Autodesk Inventor part; units mm, degrees
ref_plane "Plan de construction1" through (0, 0, 5) normal (0, 0, 1) x (1, 0, 0)
ref_plane "YZ Plane" through (0, 0, 0) normal (1, 0, 0) x (0, 1, 0)
ref_plane "XZ Plane" through (0, 0, 0) normal (0, 1, 0) x (-1, 0, 0)
sketch "Esquisse1" plane through (0, 0, 0) normal (0, 1, 0) x (-1, 0, 0)
  arc A0 (0, -5) -> (0, 5) centre (0, 0) ccw
  line L0 (0, 5) -> (0, -5)
  dimension "d1" = 5
revolve "Révolution1" add sketch "Esquisse1" angle 360 about axis through (0, 0, 5) along (0, 0, -1)
ref_plane "Plan de construction1" through (0, 0, 5) normal (0, 0, 1) x (1, 0, 0)
sketch "Esquisse2" plane through (0, 0, 5) normal (0, 0, 1) x (1, 0, 0)
  circle A0 centre (0, 0) radius 2.5
  dimension "d4" = 5
extrude "Extrusion1" cut sketch "Esquisse2" against normal blind 0.5
sketch "Esquisse3" plane through (0, 0, 4.5) normal (0, 0, 1) x (1, 0, 0)
  circle A0 centre (0, 0) radius 2.1794
hole "Perçage1" at (0, 0, 4.5) direction (0, 0, -1) diameter 3.242 depth 5.5 tip angle 118
properties part number "boule_serrage_main" material "Plastique ABS"
Geometry check sheet. Reference: the model listing, model coordinates, mm. Round coordinates to 2 decimals unless told otherwise and drop trailing zeros. Write each loop counter-clockwise with the first axis right and the second up, starting at its lowest first coordinate (ties: lowest second). Pieces come first, ordered by that corner, then holes. Notation, with made-up numbers: (39.5, 41) - (66.5, 41) arc R15 ccw to (66.5, 60) - close; hole circle Ø1 at (55, 58). An arc over 180 degrees is marked (long way). Write each question's results on one line, items separated by ' | '.
(1) Sectioned sample at B-B, the plane x = 3. Enter the section's corners in (y, z).
Computed:
outline: circle Ø8 at (0, 0)
(2) Depth check by flat-ended pin: pin 1 Ø2 at (y, z) = (-1.5, -3.5) entering from +X; pin 2 Ø2 at (x, y) = (0, 2) entering from -Z; pin 3 Ø6 at (x, y) = (2.5, 2) entering from -Z. Enter the tip coordinate at first touch or a pass-through.
Computed:
pin 1: stops at x = 4.14 | pin 2: stops at z = -4.9 | pin 3: stops at z = -5
(3) Sectioned sample at A-A, the plane y = -4. Enter the section's corners in (x, z), plus the area to 3 significant figures.
Computed:
outline: circle Ø6 at (0, 0) | area: 28.3 mm^2
(4) Sectioned sample at C-C, the plane z = 2.25. Enter the section's corners in (x, y).
Computed:
outline: circle Ø8.93 at (0, 0); hole circle Ø3.24 at (0, 0)
(5) Draft check along X on faces 1 (the face through (0, 2, 4.5)), 2 (the face through (-0.275, 0.061, -1.805)). Enter one of: pulls with the +X half, pulls with the -X half, needs draft (parallel to the pull), parting line crosses it, or undercut.
Computed:
face 1: needs draft | face 2: undercut
(6) Thickness scan on probe 1 along Y at (x, z) = (0, 0.45); probe 2 along Y at (x, z) = (0.25, 1.5); probe 3 along X at (y, z) = (1, -0.75). Record the ranges inside material, lowest first. Write a range as from..to.
Computed:
probe 1: y = -4.98..-1.62, 1.62..4.98 | probe 2: y = -4.76..-1.6, 1.6..4.76 | probe 3: x = -4.84..-1.28, 1.28..4.84
